Autodesk Inventor part; units mm, degrees
ref_plane "YZ Plane" through (0, 0, 0) normal (1, 0, 0) x (0, 1, 0)
ref_plane "XZ Plane" through (0, 0, 0) normal (0, 1, 0) x (-1, 0, 0)
ref_plane "XY Plane" through (0, 0, 0) normal (0, 0, 1) x (1, 0, 0)
sketch "Szkic1" plane through (0, 0, 0) normal (0, 1, 0) x (-1, 0, 0)
  circle A0 centre (0, 0) radius 2.5
  line L0 (-5, 5) -> (5, 5)
  line L1 (5, 5) -> (5, -5)
  line L2 (5, -5) -> (-5, -5)
  line L3 (-5, -5) -> (-5, 5)
  line L4 (-5, 5) -> (5, -5) construction
  line L5 (5, 5) -> (-5, -5) construction
  circle A1 centre (0, 0) radius 2
  dimension "d0" = 5
  dimension "d1" = 10
  dimension "d2" = 10
  dimension "d7" = 4
extrude "Wyciągnięcie proste1" add sketch "Szkic1" along normal blind 0.6 contours L0 L1 L2 L3
extrude "Wyciągnięcie proste2" add sketch "Szkic1" along normal blind 6 contours A0 | A1
extrude "Wyciągnięcie proste3" add sketch "Szkic1" against normal blind 0.4 contours A1
fillet "Zaokrąglenie1" radius 2 1 edges at (2, -0.4, 0)
chamfer "Faza1" distance 3 angle 45 4 edges at (-5, 0.3, 5) (5, 0.3, 5) (5, 0.3, -5) (-5, 0.3, -5)
fillet "Zaokrąglenie2" radius 1 1 edges at (2.5, 6, 0)
properties part number "button"
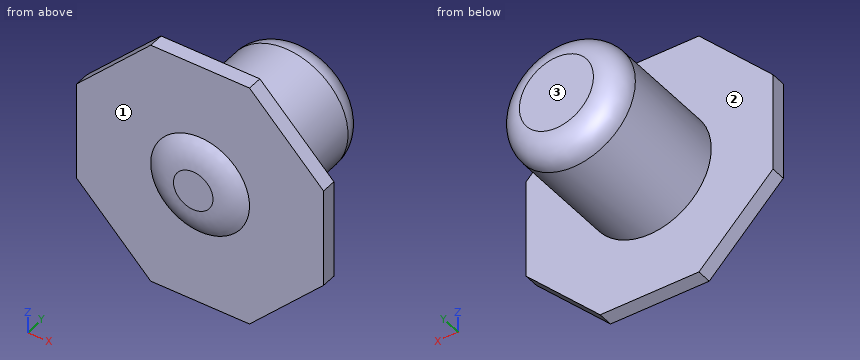
The listing builds one solid part. Answer for the finished solid, in the listing's coordinates (mm). Face numbers are marked on the shaded views. A direction names the side the tool comes from. Give positions to 0.01 mm unless a question says otherwise; leave off trailing zeros. Write each loop counter-clockwise with the first axis right and the second up, starting at its lowest first coordinate (ties: lowest second). Pieces come first, ordered by that corner, then holes.
1) Section C-C (y = 1) is taken. Write down the section's boundary in (x, z).
2) Find the intervals of material crossed by L1, parallel to Y at x = -0.25, z = 3; L2, parallel to Z at x = -0.5, y = 3.5; L3, parallel to X at y = 5.25, z = -2, in increasing order.
3) Section B-B (x = 4) is taken. Write down the section's boundary in (y, z), and give its area (3 significant figures).
4) Given P1, Ø2, axis at x = -3, y = 5.5, coming from the -Z side; P2, Ø3, axis at x = 0, z = 1, coming from the -Y side; P3, Ø1, axis at x = 2.5, z = -1, coming from the -Y side, each flat-ended and moving along its own axis, determine where each tip first touches the part or whether it passes through.
5) A tool of negligible diameter and unlimited length cuts with its end or side. For the marked faces 1, 2 and 3, from which of +Z, -Z, +X, -X, +Y, -Y can it reach the whole face along a straight path? Write none if from no direction.
6) Section A-A (z = 3.25) is taken. Write down the section's boundary in (x, y).
Response:
1. outline: circle Ø5 at (0, 0)
2. L1: y = 0 to 0.6
2. L2: z = -2.45 to 2.45
2. L3: x = -1.45 to 1.45
3. outline: (0, -3) - (0.6, -3) - (0.6, 3) - (0, 3) - close
3. area: 3.60 mm2
4. P1: stops at z = -1.4
4. P2: stops at y = -0.4
4. P3: stops at y = 0
5. face 1: -Y
5. face 2: +Y
5. face 3: +Z, -Z, +X, -X, +Y
6. outline: (-3.75, 0) - (3.75, 0) - (3.75, 0.6) - (-3.75, 0.6) - close
